Autodesk Fusion 360 part; units mm, degrees
sketch "Sketch1" plane through (0, 0, 0) normal (0, 0, 1) x (1, 0, 0) in component "Box"
  line L0 (88.9, -50.8) -> (-88.9, -50.8)
  line L1 (-101.6, -38.1) -> (-101.6, 38.1)
  line L2 (-88.9, 50.8) -> (88.9, 50.8)
  line L3 (101.6, 38.1) -> (101.6, -38.1)
  line L4 (101.6, -50.8) -> (-101.6, 50.8) construction
  line L5 (-101.6, -50.8) -> (101.6, 50.8) construction
  arc A0 (-88.9, 50.8) -> (-101.6, 38.1) centre (-88.9, 38.1) ccw
  arc A1 (101.6, 38.1) -> (88.9, 50.8) centre (88.9, 38.1) ccw
  arc A2 (88.9, -50.8) -> (101.6, -38.1) centre (88.9, -38.1) ccw
  arc A3 (-101.6, -38.1) -> (-88.9, -50.8) centre (-88.9, -38.1) ccw
  arc A4 (111.76, 38.1) -> (88.9, 60.96) centre (88.9, 38.1) ccw
  line L6 (-88.9, 60.96) -> (88.9, 60.96)
  arc A5 (-88.9, 60.96) -> (-111.76, 38.1) centre (-88.9, 38.1) ccw
  line L7 (-111.76, -38.1) -> (-111.76, 38.1)
  arc A6 (-111.76, -38.1) -> (-88.9, -60.96) centre (-88.9, -38.1) ccw
  line L8 (88.9, -60.96) -> (-88.9, -60.96)
  arc A7 (88.9, -60.96) -> (111.76, -38.1) centre (88.9, -38.1) ccw
  line L9 (111.76, 38.1) -> (111.76, -38.1)
  dimension "d1" = 203.2
  dimension "d2" = 101.6
  dimension "d3" = 12.7
  dimension "d4" = -10.16
extrude "Extrude1" add sketch "Sketch1" along normal blind 50.8 makes body 1 in component "Screew"
copy_body "CutPasteBodies1" bodies 1 removing the originals makes body 2 in component "Box"
extrude "Extrude1'" add sketch "Sketch1" along normal blind 10.16 contours L0 L1 L2 L3 A0 A1 A2 A3 bodies 2 in component "Box"
sketch "Sketch1 (1)" plane through (0, 0, 10.16) normal (0, 0, 1) x (-1, 0, 0) in component "Box"
  arc A0 (88.9, -50.8) -> (101.6, -38.1) centre (88.9, -38.1) ccw
  line L0 (101.6, -38.1) -> (101.6, 38.1)
  arc A1 (101.6, 38.1) -> (88.9, 50.8) centre (88.9, 38.1) ccw
  line L1 (88.9, 50.8) -> (-88.9, 50.8)
  arc A2 (-88.9, 50.8) -> (-101.6, 38.1) centre (-88.9, 38.1) ccw
  line L2 (-101.6, 38.1) -> (-101.6, -38.1)
  arc A3 (-101.6, -38.1) -> (-88.9, -50.8) centre (-88.9, -38.1) ccw
  line L3 (-88.9, -50.8) -> (88.9, -50.8)
  line L4 (100.33, 52.07) -> (-100.33, 52.07)
  line L5 (-100.33, 52.07) -> (-100.33, -52.07)
  line L6 (-100.33, -52.07) -> (100.33, -52.07)
  line L7 (100.33, -52.07) -> (100.33, 52.07)
  line L8 (100.33, 52.07) -> (-100.33, -52.07) construction
  line L9 (-100.33, 52.07) -> (100.33, -52.07) construction
  dimension "d9" = 200.66
  dimension "d10" = 104.14
hole "Hole1" at (100.33, 52.07, 10.16) at (100.33, -52.07, 10.16) at (-100.33, -52.07, 10.16) at (-100.33, 52.07, 10.16) direction (0, 0, -1) diameter 6.57 depth 25.4 tip angle 118 bodies 2 in component "Box"
component "Lid" placed x (1, 0, 0) y (0, 1, 0) z (0, 0, 1) at (0, 0, 0)
component "Box" placed x (1, 0, 0) y (0, 1, 0) z (0, 0, 1) at (0, 0, 0)
component "Screew" placed x (1, 0, 0) y (0, 1, 0) z (0, 0, 1) at (0, 0, 0)
The model under review builds one solid part; all positions refer to its coordinate system, in mm. A direction names the side the tool comes from. Round coordinates to 2 decimals unless told otherwise and drop trailing zeros. Write each loop counter-clockwise with the first axis right and the second up, starting at its lowest first coordinate (ties: lowest second). Pieces come first, ordered by that corner, then holes. Notation, with made-up numbers: M -28,0.5 L -23,0.5 A21 ccw -23,39.5 Z; hole C -9.75,-37 d2. An arc over 180 degrees is marked long. Answer as CSV lines item,"result". Start each with the question number.
Q1. Consider section A-A, the plane z = 47.5. Give the boundary of the cut face in (x, y).
Q2. Consider section C-C, the plane y = 27. Give the boundary of the cut face in (x, z), then the cut area to 3 significant figures.
Q3. Consider section B-B, the plane x = 22.5. Give the boundary of the cut face in (y, z).
Q4. The part is to be moulded in two halves that separate along Y. For faces 4 (the face through (-1, -54, 50.8)), 5 (the face through (-97.98, 46.98, 30.2)), 6 (the face through (-1, 60.96, 25)), 7 (the face through (-104.886, -54.441, 25.044)), say which applies: +Y half, -Y half, draft (parallel to the pull), parting line (faces both ways), or undercut.
Q5. Tool access review of faces 1 (the face through (1, -50.8, 30)), 2 (the face through (-103.587, 52.498, 5.009)), 3 (the face through (105.241, -54.086, 25.044)): name each direction out of +Z, -Z, +X, -X, +Y, -Y from which nothing blocks a thin tool from reaching the whole face with its end or side.
Q6. Clearance check with flat-ended pins moving along their axes: P1, Ø2, axis at x = 99.5, y = -52.5, coming from the -Z side; P2, Ø6, axis at y = -44.5, z = 14, coming from the -X side; P3, Ø12, axis at y = -44.5, z = 9, coming from the +X side. State where each tip first meets the part, or that it passes through.
Q7. Wall thickness on line 1 along Y through (x, z) = (35, 34); line 2 along X through (y, z) = (-26, 25.5); line 3 along X through (y, z) = (52, 7): over which ranges is each line inside the solid? List them lowest first.
Result set:
1,outline,"M -111.76,-38.1 A22.86 ccw -88.9,-60.96 L 88.9,-60.96 A22.86 ccw 111.76,-38.1 L 111.76,38.1 A22.86 ccw 88.9,60.96 L -88.9,60.96 A22.86 ccw -111.76,38.1 Z; hole M -101.6,-38.1 A12.7 ccw -88.9,-50.8 L 88.9,-50.8 A12.7 ccw 101.6,-38.1 L 101.6,38.1 A12.7 ccw 88.9,50.8 L -88.9,50.8 A12.7 ccw -101.6,38.1 Z"
2,outline,"M -111.76,0 L 111.76,0 L 111.76,50.8 L 101.6,50.8 L 101.6,10.16 L -101.6,10.16 L -101.6,50.8 L -111.76,50.8 Z"
2,area,"3,100 mm²"
3,outline,"M -60.96,0 L 60.96,0 L 60.96,50.8 L 50.8,50.8 L 50.8,10.16 L -50.8,10.16 L -50.8,50.8 L -60.96,50.8 Z"
4,face 4,"draft"
4,face 5,"undercut"
4,face 6,"+Y half"
4,face 7,"-Y half"
5,face 1,"+Z"
5,face 2,"-Z"
5,face 3,"+Z, -Z, +X, -Y"
6,P1,"stops at z = 10.16"
6,P2,"stops at x = -111.51"
6,P3,"stops at x = 111.76"
7,line 1,"y = -60.96 to -50.8, 50.8 to 60.96"
7,line 2,"x = -111.76 to -101.6, 101.6 to 111.76"
7,line 3,"x = -107.05 to -103.61, -97.05 to 97.05, 103.61 to 107.05"
